Solid Edge part; units mm, degrees
sketch "Sketch1" plane through (0, 0, 0) normal (1, 0, 0) x (0, 1, 0)
  line L0 (25, 75) -> (25, 25)
  line L1 (25, 25) -> (0, 25)
  line L2 (0, 0) -> (0, 25)
  line L3 (0, 0) -> (12, 0)
  line L4 (12, 0) -> (12, 9)
  line L5 (12, 9) -> (51, 9)
  line L6 (51, 9) -> (51, 0)
  line L7 (51, 0) -> (63, 0)
  line L8 (63, 0) -> (63, 75)
  line L9 (63, 75) -> (25, 75)
extrude "Protrusion1" add sketch "Sketch1" against normal blind 100
sketch "Sketch2" plane through (-50, 44, 75) normal (0, 0, 1) x (1, 0, 0)
  line L0 (25, 0) -> (25, -19)
  line L1 (-25, 0) -> (25, 0)
  line L2 (-25, -19) -> (-25, 0)
extrude "ExtrudedCutout_2" cut sketch "Sketch2" against normal blind 38 material side at (-25.05, 34.5, 75)
sketch "Sketch3" plane through (-50, 12.5, 25) normal (0, 0, 1) x (1, 0, 0)
  line L0 (18, -12.5) -> (18, 12.5)
  line L1 (18, 12.5) -> (-18, 12.5)
  line L2 (-18, -12.5) -> (-18, 12.5)
extrude "ExtrudedCutout_3" cut sketch "Sketch3" against normal blind 71.1799 material side at (-32.05, 12.5, 25)
Build history of the part. All positions in model axes, mm. A direction names the side the tool comes from. Coordinates: 2 decimals unless noted, no trailing zeros. Order: outer loops, then holes, each group sorted by start corner. A loop starts at its lowest first (then second) coordinate and runs counter-clockwise, first axis right, second up. Notation, with made-up numbers: (22.5, -29.75) -> (75.5, -29.75) arc R19 cw to (75.5, -23.75) -> close; hole circle Ø1 at (-8, 49.25). An arc over 180 degrees is marked (long way). One line per item, written item: value.
(1) Slice it at B-B, the plane y = 10. List the corners of the cut face in (x, z).
Checked values:
outline: (-100, 0) -> (-68, 0) -> (-68, 25) -> (-100, 25) -> close; (-32, 0) -> (0, 0) -> (0, 25) -> (-32, 25) -> close
(2) Tool access for faces 4 (the flat face through (-84, 13, 25)), 5 (the flat face through (-49, 51, 5)), 6 (the flat face through (-75, 34, 56)), 7 (the flat face through (-32, 12, 15)): list every direction of +Z, -Z, +X, -X, +Y, -Y with a clear straight run to the whole face (end or side of a thin tool).
Checked values:
face 4: +Z, +X, -X, -Y
face 5: -Z, +X, -X
face 6: +Z, -Y
face 7: +Z, -Z, -Y
(3) Probe line 1 (X direction, y = 17, z = 14.5); line 2 (X direction, y = 26, z = 66.5); line 3 (Y direction, x = -6.5, z = 44). List the from-to ranges inside material, lowest first. Write a range as [from, to].
Checked values:
line 1: [-100, -68], [-32, 0]
line 2: [-100, -75], [-25, 0]
line 3: [25, 63]
(4) Mould opens along Y. For faces 1 (the flat face through (-84, 0, 12)), 2 (the flat face through (0, 38, 37)), 3 (the flat face through (-49, 31, 9)) say: pulls with the +Y half, pulls with the -Y half, needs draft (parallel to the pull), parting line crosses it, or undercut.
Checked values:
face 1: pulls with the -Y half
face 2: needs draft
face 3: undercut
(5) Slice it at A-A, the plane z = 5.5. List the corners of the cut face in (x, y).
Checked values:
outline: (-100, 0) -> (-68, 0) -> (-68, 12) -> (-100, 12) -> close; (-100, 51) -> (0, 51) -> (0, 63) -> (-100, 63) -> close; (-32, 0) -> (0, 0) -> (0, 12) -> (-32, 12) -> close
(6) Slice it at D-D, the plane z = 70. List the corners of the cut face in (x, y).
Checked values:
outline: (-100, 25) -> (-75, 25) -> (-75, 44) -> (-25, 44) -> (-25, 25) -> (0, 25) -> (0, 63) -> (-100, 63) -> close
(7) Drop flat-ended pins along their axis: pin 1 Ø7.5 at (x, y) = (-16, 14.5) entering from +Z; pin 2 Ø7 at (x, z) = (-60.5, 4) entering from -Y; pin 3 Ø20 at (x, z) = (-57.5, 48.5) entering from -Y. Give the stop position or say it passes through.
Checked values:
pin 1: z = 25
pin 2: y = 51
pin 3: y = 44
(8) Slice it at C-C, the plane x = -70. List the corners of the cut face in (y, z), plus the area to 3 significant figures.
Checked values:
outline: (0, 0) -> (12, 0) -> (12, 9) -> (51, 9) -> (51, 0) -> (63, 0) -> (63, 75) -> (44, 75) -> (44, 37) -> (25, 37) -> (25, 25) -> (0, 25) -> close
area: 2,400 mm2
